from build123d import *

# Parameters (mm, degrees)
CHAMFER1_SIZE = 1


with BuildPart() as part:
    # Sketch1 → Revolve1 (revolve)
    with BuildSketch(Plane.XY, mode=Mode.PRIVATE) as revolve1_sk:
        Polygon((0, 0), (0, 4), (3.1, 4), (3.1, 3), (4, 3), (4, 4), (40, 4), (40, 3), (40.9, 3), (40.9, 4), (44, 4), (44, 0), align=None)
    revolve(revolve1_sk.sketch.rotate(Axis((0, 0, 0), (1, 0, 0)), 90), axis=Axis((0, 0, 0), (1, 0, 0)))

    # Chamfer1
    chamfer1_edges = [part.edges().sort_by_distance(p)[0] for p in [
        (0, 0, -4),
        (44, 0, -4),
    ]]
    chamfer(chamfer1_edges, length=CHAMFER1_SIZE)


solid = part.part
The listing builds one solid part. Answer for the finished solid, in the listing's coordinates (mm). A direction names the side the tool comes from. Coordinates: 2 decimals unless noted, no trailing zeros. Write each loop counter-clockwise with the first axis right and the second up, starting at its lowest first coordinate (ties: lowest second). Pieces come first, ordered by that corner, then holes. Notation, with made-up numbers: (36.5, 85) -> (46.5, 85) arc R26 ccw to (46.5, 110) -> close; hole circle Ø1 at (27.25, -33). An arc over 180 degrees is marked (long way). One line per question, with ' | ' between items.
1. Section A-A (z = 0) is taken. Determine the outline of the cut face in (x, y), and give its area (3 significant figures).
Verdict:
outline: (0, -3) -> (1, -4) -> (3.1, -4) -> (3.1, -3) -> (4, -3) -> (4, -4) -> (40, -4) -> (40, -3) -> (40.9, -3) -> (40.9, -4) -> (43, -4) -> (44, -3) -> (44, 3) -> (43, 4) -> (40.9, 4) -> (40.9, 3) -> (40, 3) -> (40, 4) -> (4, 4) -> (4, 3) -> (3.1, 3) -> (3.1, 4) -> (1, 4) -> (0, 3) -> close | area: 346 mm^2
2. Straight lines are drawn through the part: line 1 (X direction, y = 2.25, z = 2.5); line 2 (X direction, y = 2.5, z = 3); line 3 (Y direction, x = 10, z = 0.25). For each, find the intervals that lie inside material, in ascending order.
Verdict:
line 1: x = 0.36 to 3.1, 4 to 40, 40.9 to 43.64 | line 2: x = 0.91 to 3.1, 4 to 40, 40.9 to 43.09 | line 3: y = -3.99 to 3.99
3. Which of the six approach directions +Z, -Z, +X, -X, +Y, -Y give full straight-line access (tool end or side, diameter ignored) to faces 1 (the flat face through (44, 0, 0)), 2 (the flat face through (4, -3, -1))?
Verdict:
face 1: +Z, -Z, +X, +Y, -Y | face 2: none
4. Section D-D (z = -3.5) is taken. State how many separate pieces and enclosed holes the cut face has, and give its area (3 significant figures).
Verdict:
separate pieces: 3 | enclosed holes: 0 | area: 158 mm^2
5. Section C-C (x = 15) is taken. Determine the outline of the cut face in (y, z).
Verdict:
outline: circle Ø8 at (0, 0)
6. Given pin 1 Ø2 at (x, y) = (10.5, 2.5) entering from -Z; pin 2 Ø1.5 at (x, y) = (24, -2.5) entering from +Z, each flat-ended and moving along its own axis, determine where each tip first touches the part or whether it passes through.
Verdict:
pin 1: stops at z = -3.71 | pin 2: stops at z = 3.6
